from build123d import *

# Parameters (mm, degrees)
BOSS_EXTRUDE1_DEPTH = 12.7
SKETCH2_W           = 557.099300044
SKETCH2_H           = 6.35
CUT_EXTRUDE1_DEPTH  = 6.35


with BuildPart() as part:
    # Sketch1 → Boss-Extrude1 (new body)
    with BuildSketch(Plane(origin=(0, 0, 0), x_dir=(0, 0, -1), z_dir=(1, 0, 0))):
        Polygon((520.7, 25.4), (533.4, 25.4), (533.4, 38.1), (520.7, 38.1), (520.7, 50.8), (533.4, 50.8), (533.4, 63.5), (520.7, 63.5), (520.7, 76.2), (533.4, 76.2), (533.4, 88.9), (520.7, 88.9), (520.7, 101.6), (12.7, 101.6), (12.7, 88.9), (0, 88.9), (0, 76.2), (12.7, 76.2), (12.7, 63.5), (0, 63.5), (0, 50.8), (12.7, 50.8), (12.7, 38.1), (0, 38.1), (0, 25.4), (12.7, 25.4), (12.7, 12.7), (0, 12.7), (0, 0), (533.4, 0), (533.4, 12.7), (520.7, 12.7), align=None)
    extrude(amount=BOSS_EXTRUDE1_DEPTH)

    # Sketch2 → Cut-Extrude1 (cut)
    with BuildSketch(Plane(origin=(0, 0, 0), x_dir=(0, 0, -1), z_dir=(1, 0, 0))):
        with Locations((263.077138041, 15.875)):
            Rectangle(SKETCH2_W, SKETCH2_H)
    extrude(amount=CUT_EXTRUDE1_DEPTH, mode=Mode.SUBTRACT)


solid = part.part
The model under review builds one solid part; all positions refer to its coordinate system, in mm. A direction names the side the tool comes from. Round coordinates to 2 decimals unless told otherwise and drop trailing zeros. Loops run counter-clockwise (first coordinate to the right, second up) from the corner with the lowest first, then second, coordinate; pieces in that order, holes last. Notation, with made-up numbers: (-8, 80) -> (-1, 80) arc R23 ccw to (-1, 104) -> close; hole circle Ø2 at (-29.5, 3). An arc over 180 degrees is marked (long way). One line per question, with ' | ' between items. Start each with the question number.
Item 1: Add section C-C, the plane y = 43. Write out the cut boundary in (x, z).
Item 2: Add section A-A, the plane z = -376.5. Write out the cut boundary in (x, y).
Item 3: Draft analysis for pull direction Y (two halves, no side actions). For faces 1 (the face through (6, 57, -533.4)), 2 (the face through (6, 63.5, -527)), 3 (the face through (6, 0, -263)), state which applies: +Y half, -Y half, draft (parallel to the pull), parting line (faces both ways), or undercut.
Item 4: Machinability: for faces 4 (the face through (6, 83, 0)), 5 (the face through (6, 70, -520.7)), 6 (the face through (6, 95, -520.7)), 7 (the face through (6, 38.1, -6)), which of the approach directions +Z, -Z, +X, -X, +Y, -Y give a long, thin tool a straight path to every point of the face, cutting with its end or side? Answer none if there is none.
Item 5: Wall thickness on line 1 along Y through (x, z) = (2.25, -34); line 2 along X through (y, z) = (19, -130); line 3 along Z through (x, y) = (12.25, 91): over which ranges is each line inside the solid? List them lowest first. Write a range as [from, to].
Item 6: For pin 1 (4 mm diameter, centred on x = 5.5, y = 67, fed in from -Z); pin 2 (4 mm diameter, centred on x = 4.5, z = -8, fed in from +Y), all flat-tipped, find the tip position at first contact; note any pin that passes through.
Return value:
1) outline: (0, -520.7) -> (12.7, -520.7) -> (12.7, -12.7) -> (0, -12.7) -> close
2) outline: (0, 0) -> (12.7, 0) -> (12.7, 101.6) -> (0, 101.6) -> (0, 19.05) -> (6.35, 19.05) -> (6.35, 12.7) -> (0, 12.7) -> close
3) face 1: draft | face 2: undercut | face 3: -Y half
4) face 4: +Z, +X, -X, +Y, -Y | face 5: -Z, +X, -X | face 6: -Z, +X, -X, +Y | face 7: +Z, +X, -X
5) line 1: y = [0, 12.7], [19.05, 101.6] | line 2: x = [6.35, 12.7] | line 3: z = [-520.7, -12.7]
6) pin 1: stops at z = -520.7 | pin 2: stops at y = 88.9
